Geometry: final body of the model. Coordinates: model frame, mm. Face numbers are marked on the shaded views. A direction names the side the tool comes from. Round coordinates to 2 decimals unless told otherwise and drop trailing zeros. Loops run counter-clockwise (first coordinate to the right, second up) from the corner with the lowest first, then second, coordinate; pieces in that order, holes last. Notation, with made-up numbers: (71.25, 0.5) -> (97.25, 0.5) arc R6 ccw to (97.25, 11.5) -> close; hole circle Ø2 at (73, 67.25). An arc over 180 degrees is marked (long way). Answer in a Markdown table with one row per item.
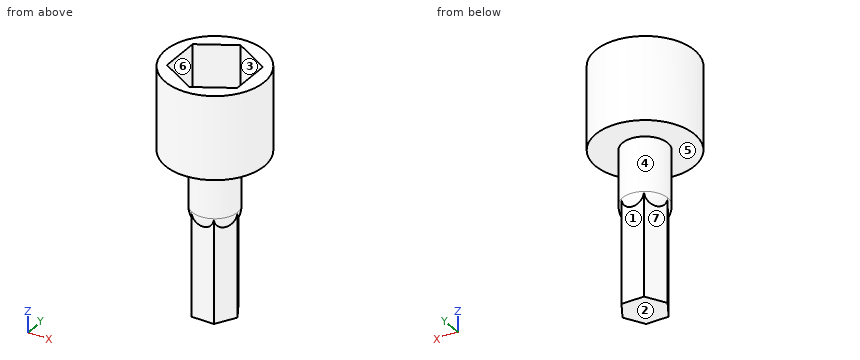
```python
from build123d import *

# Parameters (mm, degrees)
F0_R     = 7.9375
F1_DEPTH = 13.335
F3_DEPTH = 8.636
F5_DEPTH = 25.4


with BuildPart() as f1:
    # F0 (on Top) → F1 (new body)
    with BuildSketch(Plane.XY):
        Circle(F0_R)
    extrude(amount=F1_DEPTH)

    # F2 (on face) → F3 (cut)
    with BuildSketch(Plane.XY.offset(13.335)):
        Polygon((5.6515, -3.262895), (5.6515, 3.262895), (0, 6.52579), (-5.6515, 3.262895), (-5.6515, -3.262895), (0, -6.52579), align=None)
    extrude(amount=-F3_DEPTH, mode=Mode.SUBTRACT)

    # F4 (on face) → F5 (join)
    with BuildSketch(Plane(origin=(0, 0, 0), x_dir=(1, 0, 0), z_dir=(0, 0, -1))):
        Polygon((-1.81109, -3.1369), (1.81109, -3.1369), (3.62218, 0), (1.81109, 3.1369), (-1.81109, 3.1369), (-3.62218, 0), align=None)
    extrude(amount=F5_DEPTH)

    # F6 (on Front) → F7 (revolve)
    with BuildSketch(Plane.XZ):
        with BuildLine():
            Line((0, 0), (-3.62218, 0))
            Line((-3.62218, 0), (-3.62218, -8.7122))
            ThreePointArc((-3.62218, -8.7122), (-2.561268, -11.273468), (0, -12.33438))
            Line((0, -12.33438), (0, 0))
        make_face()
    revolve(axis=Axis((0, 0, -6.16719), (0, 0, -1)))


solid = f1.part
```
Item 1: Pin query (flat end, axial travel): pin 1 Ø1.1 at (x, z) = (0.5, -13.5) entering from -Y; pin 2 Ø5 at (y, z) = (-1, 8) entering from +X; pin 3 Ø1 at (x, z) = (-3.5, 7) entering from -Y; pin 4 Ø2 at (y, z) = (-3, 3.5) entering from +X. Return the tip coordinate at first contact, or that it passes through.
Answer:
| item | result |
|---|---|
| pin 1 | stops at y = -3.14 |
| pin 2 | stops at x = 7.94 |
| pin 3 | stops at y = -7.35 |
| pin 4 | stops at x = 7.68 |
Item 2: Cut plane B-B (x = 4). Output: boundary loops of the cut face in (y, z) (3 decimals).
Answer:
| item | result |
|---|---|
| outline | (-6.856, 0) -> (6.856, 0) -> (6.856, 13.335) -> (4.216, 13.335) -> (4.216, 4.699) -> (-4.216, 4.699) -> (-4.216, 13.335) -> (-6.856, 13.335) -> close |
Item 3: Cut plane D-D (z = -18). Output: boundary loops of the cut face in (x, y), then the cut area to 3 significant figures.
Answer:
| item | result |
|---|---|
| outline | (-3.62, 0) -> (-1.81, -3.14) -> (1.81, -3.14) -> (3.62, 0) -> (1.81, 3.14) -> (-1.81, 3.14) -> close |
| area | 34.1 mm² |
Item 4: Line query: probe 1 along Y at (x, z) = (0, 12); probe 2 along Z at (x, y) = (5.25, -5.5) (3 decimals); probe 3 along Z at (x, y) = (-2.75, -0.75). Output: solid intervals per line, ascending. Write a range as [from, to].
Answer:
| item | result |
|---|---|
| probe 1 | y = [-7.94, -6.53], [6.53, 7.94] |
| probe 2 | z = [0, 13.335] |
| probe 3 | z = [-25.4, 4.7] |
Item 5: Reachability of the marked faces 5, 6 and 7 from +Z, -Z, +X, -X, +Y, -Y: full face, straight path, thin tool, end or side. Return the list, or none.
Answer:
| item | result |
|---|---|
| face 5 | -Z |
| face 6 | +Z |
| face 7 | -Z, -X, +Y |
Item 6: Cut plane C-C (y = 5.25). Output: boundary loops of the cut face in (x, z) (3 decimals), then the cut area to 3 significant figures.
Answer:
| item | result |
|---|---|
| outline | (-5.953, 0) -> (5.953, 0) -> (5.953, 13.335) -> (2.21, 13.335) -> (2.21, 4.699) -> (-2.21, 4.699) -> (-2.21, 13.335) -> (-5.953, 13.335) -> close |
| area | 121 mm² |
Item 7: Draft query along Y for the marked faces 1, 2, 3 and 4. Return one class per face: pulls with the +Y half, pulls with the -Y half, needs draft (parallel to the pull), parting line crosses it, or undercut.
Answer:
| item | result |
|---|---|
| face 1 | pulls with the +Y half |
| face 2 | needs draft |
| face 3 | undercut |
| face 4 | parting line crosses it |
Item 8: Cut plane A-A (z = 6.5). Output: boundary loops of the cut face in (x, y) (1 decimal), then the cut area to 3 significant figures.
Answer:
| item | result |
|---|---|
| outline | circle Ø15.9 at (0, 0); hole (-5.7, -3.3) -> (0, -6.5) -> (5.7, -3.3) -> (5.7, 3.3) -> (0, 6.5) -> (-5.7, 3.3) -> close |
| area | 87.3 mm² |
